Model file for the job. Use its own axes, mm. A direction names the side the tool comes from. Give positions to 0.01 mm unless a question says otherwise; leave off trailing zeros. Write each loop counter-clockwise with the first axis right and the second up, starting at its lowest first coordinate (ties: lowest second). Pieces come first, ordered by that corner, then holes. Notation, with made-up numbers: M 81,10.25 L 115,10.25 A20 cw 115,18.25 Z; hole C 10,51.5 d11. An arc over 180 degrees is marked long. Answer as a JSON object with one key per item and string values. Group by question number.
```python
from build123d import *

# Parameters (mm, degrees)
F0_R     = 19
F1_DEPTH = 2
F2_W     = 7.969366
F2_H     = 26.664181
F3_DEPTH = 0.75
F5_R     = 19
F6_DEPTH = 2
F7_R     = 19
F7_R_2   = 18
F8_DEPTH = 5


with BuildPart() as f1:
    # F0 (on Top) → F1 (new body)
    with BuildSketch(Plane.XY):
        Circle(F0_R)
    extrude(amount=F1_DEPTH)

    # F2 (on face) → F3 (join)
    with BuildSketch(Plane.XY.offset(2)):
        with Locations((-7.822287, -0.156961)):
            Rectangle(F2_W, F2_H)
    extrude(amount=F3_DEPTH)

    # F4: F1 across face


with BuildPart() as f1_1:
    add(f1.part)
    add(f1.part.mirror(Plane(origin=(-7.822287, -0.156961, 2.75), x_dir=(1, 0, 0), z_dir=(0, 0, 1))))

    # F5 (on face) → F6 (cut)
    with BuildSketch(Plane.XY.offset(5.5)):
        Circle(F5_R)
        Polygon((-4.359122, 13.449247), (16.25054, 0), (-4.085717, -13.445996), (-11.66215, -13.445996), (-11.66215, 13.449247), align=None, mode=Mode.SUBTRACT)
    extrude(amount=-F6_DEPTH, mode=Mode.SUBTRACT)

    # F7 (on face) → F8 (join)
    with BuildSketch(Plane(origin=(0, 0, 0), x_dir=(1, 0, 0), z_dir=(0, 0, -1))):
        Circle(F7_R)
        Circle(F7_R_2, mode=Mode.SUBTRACT)
    extrude(amount=F8_DEPTH)


solid = f1_1.part
```
Q1. Slice it at A-A, the plane x = 0. Write the cut outline in (y, z).
Q2. Wall check: L1, parallel to Y at x = 0, z = -1.9; L2, parallel to Z at x = 7.5, y = 5.5. Give the ranges that are in metal, low to high.
Q3. Slice it at B-B, the plane z = -3. Write the cut outline in (x, y), then the cut area to 3 significant figures.
Q4. Slice it at D-D, the plane x = -9. Write the cut outline in (y, z), then the cut area to 3 significant figures.
Q5. Drop flat-ended pins along their axis: P1, Ø4, axis at y = 6.5, z = 2, coming from the -X side; P2, Ø1, axis at y = -4, z = 4.5, coming from the -X side; P3, Ø10, axis at x = 10, y = 3, coming from the -Z side. Give the stop position or say it passes through.
Q6. 3-axis set-ups, long thin cutter, end or side, ignore diameter. For faces 1 (the flat face through (5.8, 6.82, 4.51)), 2 (the flat face through (6.22, -6.63, 4.51)), 3 (the flat face through (-3.838, 0, 3)): which of +Z, -Z, +X, -X, +Y, -Y reach the whole face in a straight line?
Q7. Two-plate mould, pull along Y, no slides. Class faces 4 (the flat face through (-11.807, 0, 3)), 5 (the cylindrical face through (-2.343, -17.847, -2.465)), 6 (the flat face through (-8, -13.489, 3)): +Y half, -Y half, draft (parallel to the pull), parting line (faces both ways), or undercut.
Q8. Slice it at C-C, the plane y = 9. Write the cut outline in (x, z).
Solved:
{
 "1": {"outline": "M -19,-5 L -18,-5 L -18,0 L 18,0 L 18,-5 L 19,-5 L 19,2 L -19,2 Z; M -10.74,3.5 L 10.6,3.5 L 10.6,5.5 L -10.74,5.5 Z"},
 "2": {"L1": "y = -19 to -18, 18 to 19", "L2": "z = 0 to 2, 3.5 to 5.5"},
 "3": {"outline": "C 0,0 d38; hole C 0,0 d36", "area": "116 mm²"},
 "4": {"outline": "M -16.73,-5 L -15.59,-5 L -15.59,0 L 15.59,0 L 15.59,-5 L 16.73,-5 L 16.73,2 L 13.18,2 L 13.18,3.5 L 13.45,3.5 L 13.45,5.5 L -13.45,5.5 L -13.45,3.5 L -13.49,3.5 L -13.49,2 L -16.73,2 Z", "area": "172 mm²"},
 "5": {"P1": "stops at x = -18.46", "P2": "stops at x = -11.66", "P3": "stops at z = 0"},
 "6": {"face 1": "+Z, +X, +Y", "face 2": "+Z, +X, -Y", "face 3": "+X, +Y, -Y"},
 "7": {"face 4": "draft", "face 5": "undercut", "face 6": "-Y half"},
 "8": {"outline": "M -16.73,-5 L -15.59,-5 L -15.59,0 L 15.59,0 L 15.59,-5 L 16.73,-5 L 16.73,2 L -3.84,2 L -3.84,3.5 L 2.46,3.5 L 2.46,5.5 L -11.66,5.5 L -11.66,3.5 L -11.81,3.5 L -11.81,2 L -16.73,2 Z"}
}
